from build123d import *

# Parameters (mm, degrees)
SKETCH1_W           = 83
SKETCH1_H           = 83
SKETCH1_W_2         = 77
SKETCH1_H_2         = 77
BOSS_EXTRUDE1_DEPTH = 50
SKETCH2_W           = 100.5
SKETCH2_H           = 80.5
CUT_EXTRUDE1_DEPTH  = 5
CHAMFER1_SIZE       = 1
SKETCH3_W           = 8
SKETCH3_H           = 8
BOSS_EXTRUDE2_DEPTH = 3


with BuildPart() as part:
    # Sketch1 → Boss-Extrude1 (new body)
    with BuildSketch(Plane(origin=(0, 0, 0), x_dir=(1, 0, 0), z_dir=(0, 1, 0))):
        Rectangle(SKETCH1_W, SKETCH1_H)
        Rectangle(SKETCH1_W_2, SKETCH1_H_2, mode=Mode.SUBTRACT)
    extrude(amount=BOSS_EXTRUDE1_DEPTH)

    # Sketch2 → Cut-Extrude1 (cut)
    with BuildSketch(Plane(origin=(0, 50, 0), x_dir=(1, 0, 0), z_dir=(0, 1, 0))):
        Rectangle(SKETCH2_W, SKETCH2_H)
    extrude(amount=-CUT_EXTRUDE1_DEPTH, mode=Mode.SUBTRACT)

    # Chamfer1
    chamfer1_edges = [part.edges().sort_by_distance(p)[0] for p in [
        (-41.5, 25, -41.5),
        (41.5, 25, -41.5),
        (41.5, 25, 41.5),
        (-41.5, 25, 41.5),
    ]]
    chamfer(chamfer1_edges, length=CHAMFER1_SIZE)

    # Sketch3 → Boss-Extrude2 (add)
    with BuildSketch(Plane(origin=(0, 1, 0), x_dir=(-1, 0, 0), z_dir=(0, -1, 0))):
        with Locations((-34.5, 34.5)):
            Rectangle(SKETCH3_W, SKETCH3_H)
    extrude(amount=-BOSS_EXTRUDE2_DEPTH)


solid = part.part
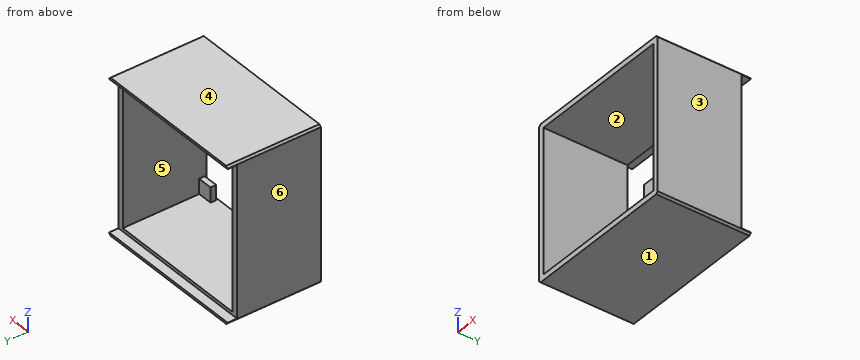
Geometry check sheet. Reference: the model listing, model coordinates, mm. Face numbers are marked on the shaded views. A direction names the side the tool comes from. Give positions to 0.01 mm unless a question says otherwise; leave off trailing zeros. Loops run counter-clockwise (first coordinate to the right, second up) from the corner with the lowest first, then second, coordinate; pieces in that order, holes last. Notation, with made-up numbers: M 11,86.5 L 38,86.5 A11 cw 38,93.5 Z; hole C 53.5,-37 d1. An arc over 180 degrees is marked long. Write each question's results on one line, items separated by ' | '.
1) Gauge pin test, flat ends, axial feed: pin 1 (4 mm diameter, centred on x = 34, z = -34.5, fed in from +Y); pin 2 (4 mm diameter, centred on x = 34, z = -33.5, fed in from -Y). Record the tip position at first contact, or that the pin passes through.
Answers follow:
pin 1: y = 4 | pin 2: y = 1
2) Section check C-C, the plane y = 13. Record the boundary of the cut face in (x, z), plus the area to 3 significant figures.
Answers follow:
outline: M -41.5,-40.5 L -40.5,-41.5 L 40.5,-41.5 L 41.5,-40.5 L 41.5,40.5 L 40.5,41.5 L -40.5,41.5 L -41.5,40.5 Z; hole M -38.5,-38.5 L 38.5,-38.5 L 38.5,38.5 L -38.5,38.5 Z | area: 958 mm2
3) Section check B-B, the plane x = -22.5. Record the boundary of the cut face in (y, z).
Answers follow:
outline: M 0,-41.5 L 50,-41.5 L 50,-40.25 L 45,-40.25 L 45,-38.5 L 0,-38.5 Z; M 0,38.5 L 45,38.5 L 45,40.25 L 50,40.25 L 50,41.5 L 0,41.5 Z
4) Section check A-A, the plane z = 11. Record the boundary of the cut face in (x, y).
Answers follow:
outline: M -41.5,0 L -38.5,0 L -38.5,45 L -41.5,45 Z; M 38.5,0 L 41.5,0 L 41.5,45 L 38.5,45 Z
5) Release check for a two-part mould opening along X. For the marked faces 3, 4, 5 and 6 record: +X half, -X half, draft (parallel to the pull), parting line (faces both ways), or undercut.
Answers follow:
face 3: +X half | face 4: draft | face 5: undercut | face 6: -X half
6) Tool access check on the marked faces 1 and 2. Record the directions out of +Z, -Z, +X, -X, +Y, -Y that give a thin tool (end or side, any length) a straight path to the whole face; none if there is none.
Answers follow:
face 1: -Z, +X, -X, +Y, -Y | face 2: +Y, -Y
7) Thickness scan on line 1 (Z direction, x = -34.5, y = 16.5). Record the ranges inside material, lowest first.
Answers follow:
line 1: -41.5 to -38.5, 38.5 to 41.5
